from build123d import *

# Parameters (mm, degrees)
EXTRUDE_1_DEPTH        = 15
SKETCH_2_W             = 180
SKETCH_2_H             = 40
EXTRUDE_2_DEPTH        = 15
PATTERN_LINEAR_1_COUNT = 4
PATTERN_LINEAR_1_PITCH = 320
SKETCH_3_R             = 4
EXTRUDE_3_DEPTH        = 1080


with BuildPart() as part:
    # 草图1 → 凸台-拉伸1 (new body)
    with BuildSketch(Plane(origin=(0, 0, 0), x_dir=(0, 0, -1), z_dir=(1, 0, 0))):
        Polygon((-90, 0), (-90, 1190), (90, 1190), (90, 0), (130, 0), (130, 1230), (-130, 1230), (-130, 0), align=None)
    extrude(amount=-EXTRUDE_1_DEPTH)

    # 草图2 → 凸台-拉伸2 (add)
    with BuildSketch(Plane(origin=(0, 0, 0), x_dir=(0, 0, -1), z_dir=(1, 0, 0))):
        with Locations((0, 90)):
            Rectangle(SKETCH_2_W, SKETCH_2_H)
    extrude_2 = extrude(amount=-EXTRUDE_2_DEPTH)

    # 阵列(线性)1: 凸台-拉伸2 ×4
    with Locations(*[(0, i * PATTERN_LINEAR_1_PITCH, 0) for i in range(1, PATTERN_LINEAR_1_COUNT)]):
        add(extrude_2)

    # 草图3 → 凸台-拉伸3 (add)
    with BuildSketch(Plane(origin=(0, 110, 0), x_dir=(1, 0, 0), z_dir=(0, 1, 0))):
        with Locations((-7.5, -35)):
            Circle(SKETCH_3_R)
    extrude_3 = extrude(amount=EXTRUDE_3_DEPTH)

    # 镜向1: 凸台-拉伸3 across plane
    add(extrude_3.mirror(Plane.XY))


solid = part.part
Model file for the job. Use its own axes, mm. Coordinates: 2 decimals unless noted, no trailing zeros. Order: outer loops, then holes, each group sorted by start corner. A loop starts at its lowest first (then second) coordinate and runs counter-clockwise, first axis right, second up. Notation, with made-up numbers: M 61,75 L 97,75 A28 cw 97,103 Z; hole C 10,62 d7. An arc over 180 degrees is marked long. Return JSON: item names as keys, results as strings.
1. Saw through at C-C (x = -7.5). Give the number of separate pieces and of enclosed holes in the cut face, and give its area (3 significant figures).
Ans:
{"separate pieces": "1", "enclosed holes": "12", "area": "150,000 mm^2"}
2. Drill centre lines: probe 1 along Y at (x, z) = (-2.25, -49.5); probe 2 along Z at (x, y) = (-7.5, 862); probe 3 along Z at (x, y) = (-9, 835). Where is each one in solid material? Low to high.
Ans:
{"probe 1": "70 to 110, 390 to 430, 710 to 750, 1030 to 1070, 1190 to 1230", "probe 2": "-130 to -90, -39 to -31, 31 to 39, 90 to 130", "probe 3": "-130 to -90, -38.71 to -31.29, 31.29 to 38.71, 90 to 130"}
3. Saw through at A-A (y = 316.5). Give the cut face in (x, z), and give its area (3 significant figures).
Ans:
{"outline": "M -15,-130 L 0,-130 L 0,-90 L -15,-90 Z; M -15,90 L 0,90 L 0,130 L -15,130 Z; C -7.5,-35 d8; C -7.5,35 d8", "area": "1,300 mm^2"}
4. Saw through at B-B (z = 9). Give the cut face in (x, y).
Ans:
{"outline": "M -15,70 L 0,70 L 0,110 L -15,110 Z; M -15,390 L 0,390 L 0,430 L -15,430 Z; M -15,710 L 0,710 L 0,750 L -15,750 Z; M -15,1030 L 0,1030 L 0,1070 L -15,1070 Z; M -15,1190 L 0,1190 L 0,1230 L -15,1230 Z"}
5. Flat gauge pin, fed straight in: pin 1 (4.5 mm diameter, centred on x = -8, z = 24.5, fed in from -Y). Where does the tip first touch, or does it go through?
Ans:
{"pin 1": "y = 70"}
